Geometry: see drawing. Coordinates: mm, zero at the bounding-box minimum. A direction names the side the tool comes from. Round coordinates to 2 decimals unless told otherwise and drop trailing zeros. Loops run counter-clockwise (first coordinate to the right, second up) from the corner with the lowest first, then second, coordinate; pieces in that order, holes last. Notation, with made-up numbers: (89, 2) - (123, 2) arc R18 cw to (123, 7) - close; hole circle Ø6 at (80, 65). An arc over 180 degrees is marked (long way). Use CSV: the item, a comma, the result in double quotes.
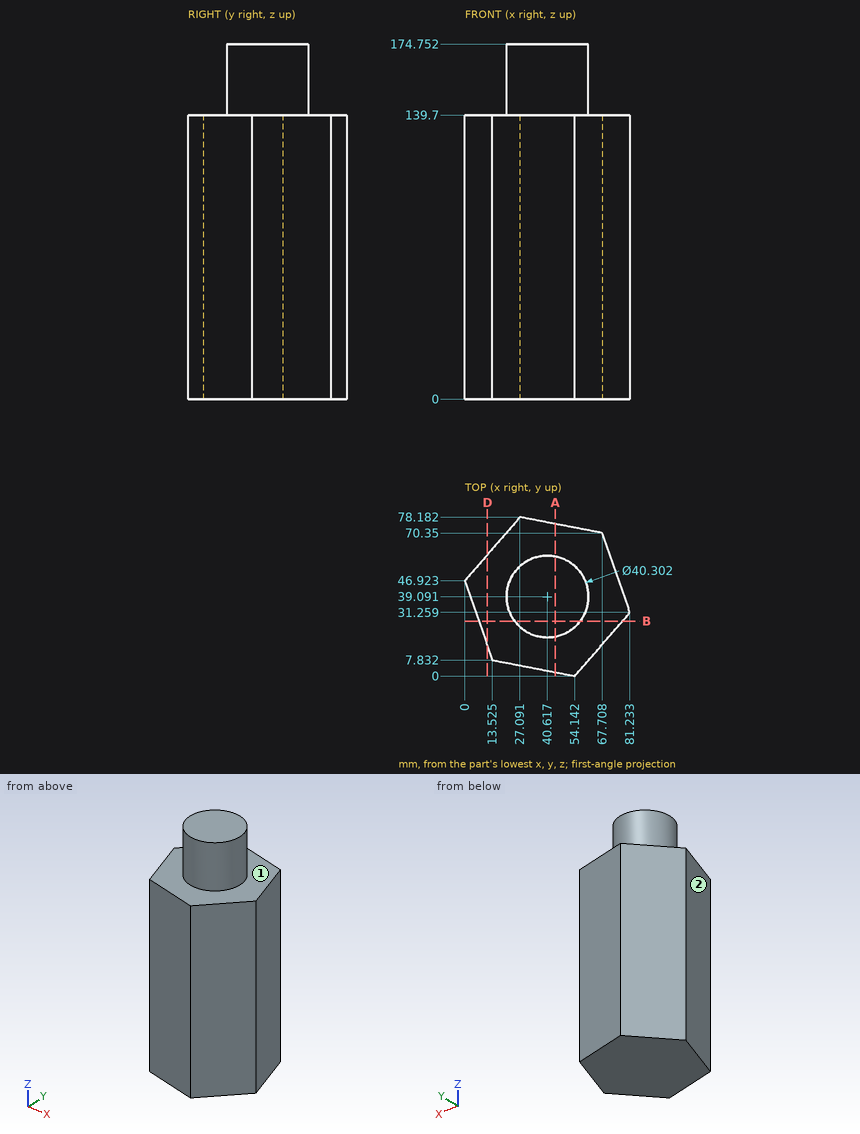
Item 1: Reachability of the marked faces 1 and 2 from +Z, -Z, +X, -X, +Y, -Y: full face, straight path, thin tool, end or side. Return the list, or none.
Final values:
face 1,"+Z"
face 2,"+Z, -Z, -X, -Y"
Item 2: Pin query (flat end, axial travel): P1, Ø1.5, axis at y = 21, z = 47.5, coming from the -X side; P2, Ø8, axis at x = 16, y = 50, coming from the +Z side; P3, Ø12, axis at y = 49.5, z = 146.5, coming from the -X side. Return the tip coordinate at first contact, or that it passes through.
Final values:
P1,"stops at x = 8.71"
P2,"stops at z = 139.7"
P3,"stops at x = 20.95"
Item 3: Section D-D on x = 11. Return the cut outline in (y, z) (1 decimal), plus the area to 3 significant figures.
Final values:
outline,"(15.1, 0) - (59.6, 0) - (59.6, 139.7) - (15.1, 139.7) - close"
area,"6,210 mm²"
Item 4: Section B-B on y = 27. Return the cut outline in (x, z) (1 decimal).
Final values:
outline,"(6.9, 0) - (77.5, 0) - (77.5, 139.7) - (56.7, 139.7) - (56.7, 174.8) - (24.5, 174.8) - (24.5, 139.7) - (6.9, 139.7) - close"
Item 5: Material intervals for line 1 (Z direction, x = 26.5, y = 67.5); line 2 (X direction, y = 20, z = 65.5) (1 decimal); line 3 (Y direction, x = 37, z = 65) (1 decimal), sorted ascending.
Final values:
line 1,"z = 0 to 139.7"
line 2,"x = 9.3 to 71.5"
line 3,"y = 3.3 to 76.3"
Item 6: Section A-A on x = 44.5. Return the cut outline in (y, z) (1 decimal), plus the area to 3 significant figures.
Final values:
outline,"(1.9, 0) - (74.8, 0) - (74.8, 139.7) - (58.9, 139.7) - (58.9, 174.8) - (19.3, 174.8) - (19.3, 139.7) - (1.9, 139.7) - close"
area,"11,600 mm²"
